```python
from build123d import *

# Parameters (mm, degrees)
SKETCH_1_R          = 2.5
EXTRUDE_1_DEPTH     = 1.7
SKETCH_2_R          = 1.5
EXTRUDE_2_DEPTH     = 14
CUT_EXTRUDE_1_DEPTH = 6.1


with BuildPart() as part:
    # 草图1 → 凸台-拉伸1 (new body)
    with BuildSketch(Plane(origin=(0, 0, 0), x_dir=(1, 0, 0), z_dir=(0, 1, 0))):
        Circle(SKETCH_1_R)
    extrude(amount=EXTRUDE_1_DEPTH)

    # 草图2 → 凸台-拉伸2 (add)
    with BuildSketch(Plane(origin=(0, 1.7, 0), x_dir=(1, 0, 0), z_dir=(0, 1, 0))):
        Circle(SKETCH_2_R)
    extrude(amount=EXTRUDE_2_DEPTH)

    # 草图3 one side → 切除-旋转3 (revolve, cut)
    with BuildSketch(Plane(origin=(0, 0, 0), x_dir=(0, 0, -1), z_dir=(1, 0, 0))):
        with BuildLine():
            ThreePointArc((2.5, 0.982204858), (1.343012135, 0.254359211), (0, 0))
            Line((0, 0), (0, -0.936416285))
            Line((0, -0.936416285), (3.543500435, -0.936416285))
            Line((3.543500435, -0.936416285), (2.5, 0.982204858))
        make_face()
    revolve(axis=Axis((0, 1.035939113, 0), (0, -1, 0)), mode=Mode.SUBTRACT)

    # 草图4 → 切除-拉伸1 (cut)
    with BuildSketch(Plane(origin=(0, -5, 0), x_dir=(1, 0, 0), z_dir=(0, 1, 0))):
        Polygon((-1, -0.2), (-0.2, -0.2), (-0.2, -1), (0.2, -1), (0.2, -0.2), (1, -0.2), (1, 0.2), (0.2, 0.2), (0.2, 1), (-0.2, 1), (-0.2, 0.2), (-1, 0.2), align=None)
    extrude(amount=CUT_EXTRUDE_1_DEPTH, mode=Mode.SUBTRACT)


solid = part.part
```
The model under review builds one solid part; all positions refer to its coordinate system, in mm. A direction names the side the tool comes from. Round coordinates to 2 decimals unless told otherwise and drop trailing zeros. Order: outer loops, then holes, each group sorted by start corner. A loop starts at its lowest first (then second) coordinate and runs counter-clockwise, first axis right, second up. Notation, with made-up numbers: (65, -15.5) -> (73, -15.5) arc R24 cw to (73, 3.5) -> close; hole circle Ø2 at (-25.75, 75). An arc over 180 degrees is marked (long way). One line per item, written item: value. Start each with the question number.
Q1. Take a section at C-C (y = 9.5). Write out the cut boundary in (x, z), and give its area (3 significant figures).
Q2. Machinability: for faces 1 (the face through (-0.6, 0.5, 0.2)), 2 (the face through (-1.5, 8.6, -0.07)), 3 (the face through (1.34, 1.34, -2.11)), which of the approach directions +Z, -Z, +X, -X, +Y, -Y give a long, thin tool a straight path to every point of the face, cutting with its end or side? Answer none if there is none.
Q3. Take a section at D-D (x = 1.3). Write out the cut boundary in (y, z).
Q4. Take a section at A-A (z = 0). Write out the cut boundary in (x, y), and give its area (3 significant figures).
Q5. Clearance check with flat-ended pins moving along their axes: pin 1 Ø0.9 at (x, y) = (-0.5, 0.5) entering from +Z; pin 2 Ø0.9 at (x, y) = (-0.5, 0.5) entering from -Z; pin 3 Ø0.9 at (y, z) = (0.5, -0.5) entering from +X. State where each tip first meets the part, or that it passes through.
Q6. Take a section at B-B (x = 0). Write out the cut boundary in (y, z), and give its area (3 significant figures).
Q7. Wall thickness on line 1 (Y direction, x = -0.15, z = 0.6); line 2 (Y direction, x = 0.55, z = 1.05); line 3 (X direction, y = 9, z = 0.1): over which ranges is each line inside the solid? List them lowest first.
Reported:
1. outline: circle Ø3 at (0, 0)
1. area: 7.07 mm2
2. face 1: -Y
2. face 2: +Y
2. face 3: +Y, -Y
3. outline: (0.98, -2.14) -> (1.7, -2.14) -> (1.7, -0.75) -> (15.7, -0.75) -> (15.7, 0.75) -> (1.7, 0.75) -> (1.7, 2.14) -> (0.98, 2.14) arc R3.43 ccw to start
4. outline: (-2.5, 0.98) arc R3.67 ccw to (-1, 0.14) -> (-1, 1.1) -> (1, 1.1) -> (1, 0.14) arc R3.67 ccw to (2.5, 0.98) -> (2.5, 1.7) -> (1.5, 1.7) -> (1.5, 15.7) -> (-1.5, 15.7) -> (-1.5, 1.7) -> (-2.5, 1.7) -> close
4. area: 46.9 mm2
5. pin 1: stops at z = 2.42
5. pin 2: stops at z = -2.42
5. pin 3: stops at x = 2.42
6. outline: (0.14, -1) arc R3.67 ccw to (0.98, -2.5) -> (1.7, -2.5) -> (1.7, -1.5) -> (15.7, -1.5) -> (15.7, 1.5) -> (1.7, 1.5) -> (1.7, 2.5) -> (0.98, 2.5) arc R3.67 ccw to (0.14, 1) -> (1.1, 1) -> (1.1, -1) -> close
6. area: 46.9 mm2
7. line 1: y = 1.1 to 15.7
7. line 2: y = 0.2 to 15.7
7. line 3: x = -1.5 to 1.5
